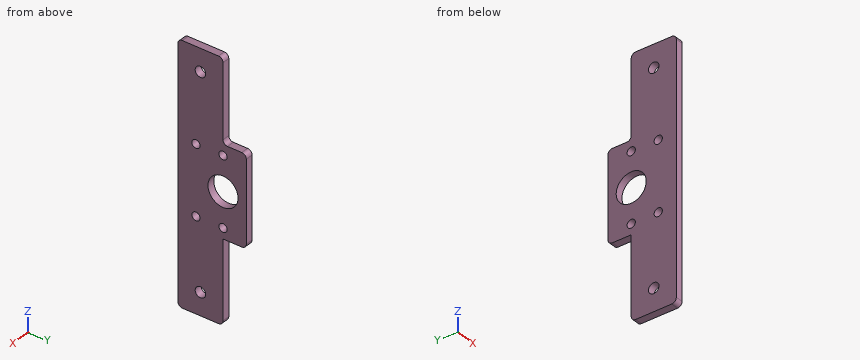
from build123d import *

# Parameters (mm, degrees)
F1_DEPTH = 5
F2_R     = 3
F3_R     = 3.5
F4_DEPTH = 5
F6_R     = 10
F6_R_2   = 2.75
F7_DEPTH = 5


# Not quite as in the source:
# - two fillets or chamfers of one size are made in one step


with BuildPart() as f1:
    # F0 (on Right) → F1 (new body)
    with BuildSketch(Plane.YZ):
        Polygon((15, 30), (15, 85), (-15, 85), (-15, -85), (15, -85), (15, -30), (30.5, -30), (30.5, 30), align=None)
    extrude(amount=F1_DEPTH)

    # F2
    f2_edges = [f1.edges().sort_by_distance(p)[0] for p in [
        (2.5, -15, 85),
        (2.5, 15, 85),
        (2.5, -15, -85),
        (2.5, 15, 30),
        (2.5, 15, -85),
        (2.5, 30.5, -30),
        (2.5, 30.5, 30),
    ]]
    fillet(f2_edges, radius=F2_R)

    # F3 (on face) → F4 (cut)
    with BuildSketch(Plane.YZ.offset(5)):
        with Locations((0, 70)):
            Circle(F3_R)
        with Locations((0, -70)):
            Circle(F3_R)
    extrude(amount=-F4_DEPTH, mode=Mode.SUBTRACT)

    # F6 (on face) → F7 (cut)
    with BuildSketch(Plane.YZ.offset(5)):
        with Locations((15, 0)):
            Circle(F6_R)
        with Locations((15, 23)):
            Circle(F6_R_2)
        with Locations((15, -23)):
            Circle(F6_R_2)
        with Locations((-3, -23)):
            Circle(F6_R_2)
        with Locations((-3, 23)):
            Circle(F6_R_2)
    extrude(amount=-F7_DEPTH, mode=Mode.SUBTRACT)


solid = f1.part
Geometry check sheet. Reference: the model listing, model coordinates, mm. Give positions to 0.01 mm unless a question says otherwise; leave off trailing zeros. Loops run counter-clockwise (first coordinate to the right, second up) from the corner with the lowest first, then second, coordinate; pieces in that order, holes last.
(1) Section check D-D on z = -43.5. Record the cut outline in (x, y), then the cut area to 3 significant figures.
From the geometry:
outline: (0, -15) - (5, -15) - (5, 15) - (0, 15) - close
area: 150 mm2
(2) Section check B-B on x = 3.85. Record the cut outline in (y, z).
From the geometry:
outline: (-15, -82) arc R3 ccw to (-12, -85) - (12, -85) arc R3 ccw to (15, -82) - (15, -30) - (27.5, -30) arc R3 ccw to (30.5, -27) - (30.5, 27) arc R3 ccw to (27.5, 30) - (18, 30) arc R3 cw to (15, 33) - (15, 82) arc R3 ccw to (12, 85) - (-12, 85) arc R3 ccw to (-15, 82) - close; hole circle Ø5.5 at (-3, -23); hole circle Ø5.5 at (-3, 23); hole circle Ø7 at (0, -70); hole circle Ø7 at (0, 70); hole circle Ø20 at (15, 0); hole circle Ø5.5 at (15, -23); hole circle Ø5.5 at (15, 23)
(3) Thickness scan on L1, parallel to Z at x = 2.85, y = -3; L2, parallel to Y at x = 4.8, z = -64; L3, parallel to Y at x = 3.85, z = -7. Record the ranges inside material, lowest first.
From the geometry:
L1: z = -85 to -71.8, -68.2 to -25.75, -20.25 to 20.25, 25.75 to 68.2, 71.8 to 85
L2: y = -15 to 15
L3: y = -15 to 7.86, 22.14 to 30.5
(4) Section check C-C on z = -4. Record the cut outline in (x, y), then the cut area to 3 significant figures.
From the geometry:
outline: (0, -15) - (5, -15) - (5, 5.83) - (0, 5.83) - close; (0, 24.17) - (5, 24.17) - (5, 30.5) - (0, 30.5) - close
area: 136 mm2
(5) Depth check by flat-ended pin: pin 1 Ø3.5 at (y, z) = (-3, 23) entering from +X; pin 2 Ø1.5 at (x, y) = (3, 21.5) entering from +Z; pin 3 Ø2.5 at (x, z) = (3, 46.5) entering from +Y. Enter the tip coordinate at first touch or a pass-through.
From the geometry:
pin 1: passes through
pin 2: stops at z = 30
pin 3: stops at y = 15
(6) Section check A-A on z = 70. Record the cut outline in (x, y).
From the geometry:
outline: (0, -15) - (5, -15) - (5, -3.5) - (0, -3.5) - close; (0, 3.5) - (5, 3.5) - (5, 15) - (0, 15) - close
